```python
from build123d import *

# Parameters (mm, degrees)
SKETCH1_R           = 9
BOSS_EXTRUDE1_DEPTH = 32
SKETCH2_W           = 40
SKETCH2_H           = 32
BOSS_EXTRUDE2_DEPTH = 11
SKETCH3_R           = 9
BOSS_EXTRUDE5_DEPTH = 11
LPATTERN1_COUNT     = 2
LPATTERN1_PITCH     = 21


with BuildPart() as part:
    # Sketch1 → Boss-Extrude1 (new body)
    with BuildSketch(Plane(origin=(0, 0, 0), x_dir=(0, 0, -1), z_dir=(1, 0, 0))):
        Circle(SKETCH1_R)
    extrude(amount=BOSS_EXTRUDE1_DEPTH)

    # Sketch2 → Boss-Extrude2 (add)
    with BuildSketch(Plane(origin=(32, 0, 0), x_dir=(0, 0, -1), z_dir=(1, 0, 0))):
        Rectangle(SKETCH2_W, SKETCH2_H)
    extrude(amount=BOSS_EXTRUDE2_DEPTH)

    # Sketch3 → Boss-Extrude5 (add)
    with BuildSketch(Plane(origin=(0, -16, 0), x_dir=(-1, 0, 0), z_dir=(0, -1, 0))):
        with BuildLine():
            Line((-43, 20), (-83, 20))
            ThreePointArc((-83, 20), (-103, 0), (-83, -20))
            Line((-83, -20), (-43, -20))
            Line((-43, -20), (-43, 20))
        make_face()
        with Locations(Location((-83, 0, 0), (0, 0, 90))):
            Circle(SKETCH3_R, mode=Mode.SUBTRACT)
    boss_extrude5 = extrude(amount=-BOSS_EXTRUDE5_DEPTH)

    # LPattern1: Boss-Extrude5 ×2
    with Locations(*[(0, i * LPATTERN1_PITCH, 0) for i in range(1, LPATTERN1_COUNT)]):
        add(boss_extrude5)


solid = part.part
```
Verification items for the finished model (mm, model axes). A direction names the side the tool comes from. Coordinates: 2 decimals unless noted, no trailing zeros. Write each loop counter-clockwise with the first axis right and the second up, starting at its lowest first coordinate (ties: lowest second). Pieces come first, ordered by that corner, then holes. Notation, with made-up numbers: M -0.75,36 L 37.25,36 A35 ccw 37.25,68 Z; hole C 82,32 d2. An arc over 180 degrees is marked long. One line per item, written item: value.
Item 1: Section check D-D, the plane z = 12. Record the boundary of the cut face in (x, y).
Check sheet entries:
outline: M 32,-16 L 99,-16 L 99,-5 L 43,-5 L 43,5 L 99,5 L 99,16 L 32,16 Z
Item 2: Gauge pin test, flat ends, axial feed: pin 1 Ø1.5 at (y, z) = (6.5, -9.5) entering from -X; pin 2 Ø2 at (y, z) = (8.5, 12.5) entering from +X; pin 3 Ø5 at (y, z) = (-10.5, -6) entering from +X; pin 4 Ø9.5 at (y, z) = (5, -1.5) entering from -X. Record the tip position at first contact, or that the pin passes through.
Check sheet entries:
pin 1: stops at x = 32
pin 2: stops at x = 99.36
pin 3: stops at x = 102.69
pin 4: stops at x = 0
Item 3: Section check B-B, the plane y = 10. Record the boundary of the cut face in (x, z), plus the area to 3 significant figures.
Check sheet entries:
outline: M 32,-20 L 83,-20 A20 ccw 83,20 L 32,20 Z; hole C 83,0 d18
area: 2,410 mm^2
Item 4: Section check C-C, the plane x = 44. Record the boundary of the cut face in (y, z).
Check sheet entries:
outline: M -16,-20 L -5,-20 L -5,20 L -16,20 Z; M 5,-20 L 16,-20 L 16,20 L 5,20 Z
Item 5: Scan lines: line 1 along Y through (x, z) = (51.5, 2.5); line 2 along Z through (x, y) = (82.5, 13); line 3 along X through (y, z) = (-8, 0). Record each from-to range of solid material in increasing order.
Check sheet entries:
line 1: y = -16 to -5, 5 to 16
line 2: z = -20 to -8.99, 8.99 to 20
line 3: x = 0 to 74, 92 to 103
Item 6: Mould release check, pull along Z, two halves, no side actions. Record for faces 4 (the flat face through (58, -7, 20)), 5 (the flat face through (68, 16, 0)), 6 (the cylindrical face through (74.214, 10.423, 1.951)): pulls with the +Z half, pulls with the -Z half, needs draft (parallel to the pull), parting line crosses it, or undercut.
Check sheet entries:
face 4: pulls with the +Z half
face 5: needs draft
face 6: undercut
Item 7: Access from +Z, -Z, +X, -X, +Y, -Y to the whole of each face (thin tool, end or side, straight path). Record for faces 1 (the cylindrical face through (15.776, 8.923, 1.172)), 2 (the flat face through (57, -7, -20)), 3 (the flat face through (43, 0, 0)).
Check sheet entries:
face 1: -X
face 2: -Z, +X, -X, +Y, -Y
face 3: +Z, -Z, +X
Item 8: Section check A-A, the plane z = 0. Record the boundary of the cut face in (x, y).
Check sheet entries:
outline: M 0,-9 L 32,-9 L 32,-16 L 74,-16 L 74,-5 L 43,-5 L 43,5 L 74,5 L 74,16 L 32,16 L 32,9 L 0,9 Z; M 92,-16 L 103,-16 L 103,-5 L 92,-5 Z; M 92,5 L 103,5 L 103,16 L 92,16 Z
